from build123d import *

# Parameters (mm, degrees)
SKETCH_1_W          = 30
SKETCH_1_H          = 27
EXTRUDE_1_DEPTH     = 1.5
SKETCH_2_R          = 0.45
SKETCH_2_W          = 0.7
SKETCH_2_H          = 0.7
CUT_EXTRUDE_1_DEPTH = 21.236106345


with BuildPart() as part:
    # Эскиз1 → Бобышка-Вытянуть1 (new body)
    with BuildSketch(Plane(origin=(0, 0, 0), x_dir=(1, 0, 0), z_dir=(0, 1, 0))):
        Rectangle(SKETCH_1_W, SKETCH_1_H)
    extrude(amount=EXTRUDE_1_DEPTH)

    # Эскиз2 → Вырез-Вытянуть1 (cut, through all)
    with BuildSketch(Plane(origin=(0, 1.5, 0), x_dir=(1, 0, 0), z_dir=(0, 1, 0))):
        with Locations(Location((-13.1, -8.72, 0), (0, 0, 270))):
            Circle(SKETCH_2_R)
        with Locations(Location((-13.1, -6.18, 0), (0, 0, 270))):
            Circle(SKETCH_2_R)
        with Locations(Location((-13.1, -3.64, 0), (0, 0, 270))):
            Circle(SKETCH_2_R)
        with Locations(Location((-13.1, -1.1, 0), (0, 0, 270))):
            Circle(SKETCH_2_R)
        with Locations(Location((-13.1, 1.44, 0), (0, 0, 270))):
            Circle(SKETCH_2_R)
        with Locations(Location((-13.1, 3.98, 0), (0, 0, 270))):
            Circle(SKETCH_2_R)
        with Locations(Location((-13.1, 6.52, 0), (0, 0, 270))):
            Circle(SKETCH_2_R)
        with Locations(Location((-13.1, 9.06, 0), (0, 0, 270))):
            Circle(SKETCH_2_R)
        with Locations(Location((-13.1, 11.6, 0), (0, 0, 270))):
            Circle(SKETCH_2_R)
        with Locations(Location((13.1, 11.6, 0), (0, 0, 90))):
            Circle(SKETCH_2_R)
        with Locations(Location((13.1, 9.06, 0), (0, 0, 90))):
            Circle(SKETCH_2_R)
        with Locations(Location((13.1, 6.52, 0), (0, 0, 90))):
            Circle(SKETCH_2_R)
        with Locations(Location((13.1, 3.98, 0), (0, 0, 90))):
            Circle(SKETCH_2_R)
        with Locations(Location((13.1, 1.44, 0), (0, 0, 90))):
            Circle(SKETCH_2_R)
        with Locations(Location((13.1, -1.1, 0), (0, 0, 90))):
            Circle(SKETCH_2_R)
        with Locations(Location((13.1, -3.64, 0), (0, 0, 90))):
            Circle(SKETCH_2_R)
        with Locations(Location((13.1, -6.18, 0), (0, 0, 90))):
            Circle(SKETCH_2_R)
        with Locations(Location((13.1, -8.72, 0), (0, 0, 90))):
            Circle(SKETCH_2_R)
        with Locations((-10.174, -11.5)):
            Rectangle(SKETCH_2_W, SKETCH_2_H)
        with Locations((-7.634, -11.5)):
            Rectangle(SKETCH_2_W, SKETCH_2_H)
        with Locations((-5.094, -11.5)):
            Rectangle(SKETCH_2_W, SKETCH_2_H)
        with Locations((-2.554, -11.5)):
            Rectangle(SKETCH_2_W, SKETCH_2_H)
        with Locations((-0.014, -11.5)):
            Rectangle(SKETCH_2_W, SKETCH_2_H)
        with Locations((2.526, -11.5)):
            Rectangle(SKETCH_2_W, SKETCH_2_H)
        with Locations((5.066, -11.5)):
            Rectangle(SKETCH_2_W, SKETCH_2_H)
        with Locations((7.606, -11.5)):
            Rectangle(SKETCH_2_W, SKETCH_2_H)
        with Locations((10.146, -11.5)):
            Rectangle(SKETCH_2_W, SKETCH_2_H)
    extrude(amount=-CUT_EXTRUDE_1_DEPTH, mode=Mode.SUBTRACT)


solid = part.part
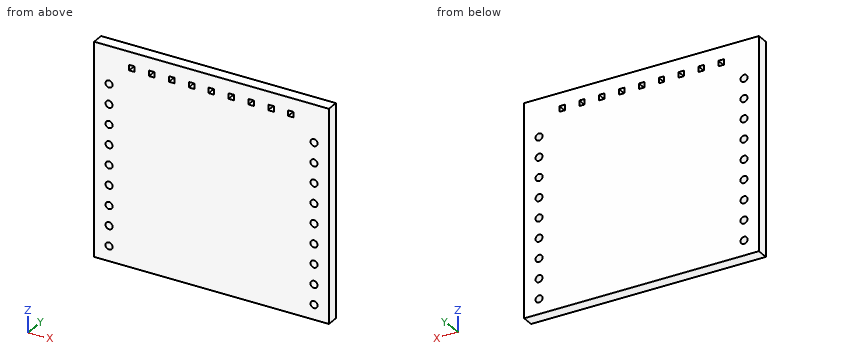
The listing builds one solid part. Answer for the finished solid, in the listing's coordinates (mm). Coordinates: 2 decimals unless noted, no trailing zeros. Order: outer loops, then holes, each group sorted by start corner. A loop starts at its lowest first (then second) coordinate and runs counter-clockwise, first axis right, second up. Notation, with made-up numbers: (66, -30) -> (94, -30) arc R31 cw to (94, 4) -> close; hole circle Ø9 at (74, -28). An arc over 180 degrees is marked (long way). Answer in a Markdown table with one row per item. Add a question column.
Item 1: Find section B-B (x = -13.1). State how many separate pieces and enclosed holes the cut face has, then the cut area to 4 significant figures.
Item 2: Find the intervals of material crossed by L1, parallel to X at y = 0.4, z = 8.72; L2, parallel to Z at x = -7.5, y = 0.1, in increasing order. Write a range as from..to.
Item 3: Find section A-A (z = -3.98). Write down the section's boundary in (x, y).
Result set:
| question | item | result |
|---|---|---|
| 1 | separate pieces | 10 |
| 1 | enclosed holes | 0 |
| 1 | area | 28.35 mm² |
| 2 | L1 | x = -15..-13.55, -12.65..12.65, 13.55..15 |
| 2 | L2 | z = -13.5..11.15, 11.85..13.5 |
| 3 | outline | (-15, 0) -> (-13.55, 0) -> (-13.55, 1.5) -> (-15, 1.5) -> close; (-12.65, 0) -> (12.65, 0) -> (12.65, 1.5) -> (-12.65, 1.5) -> close; (13.55, 0) -> (15, 0) -> (15, 1.5) -> (13.55, 1.5) -> close |
